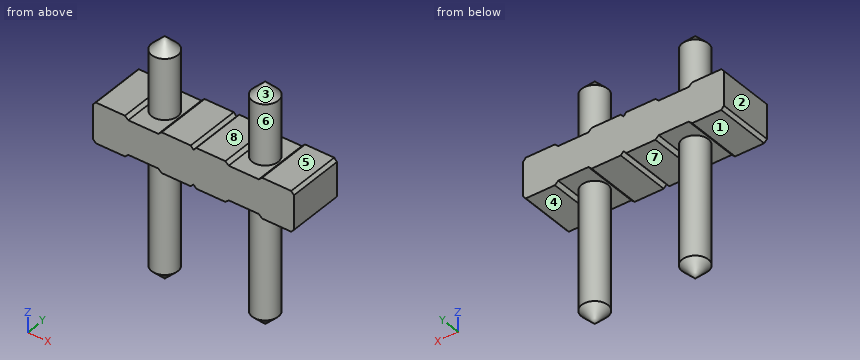
```python
from build123d import *

# Parameters (mm, degrees)
BOSS_EXTRUDE1_DEPTH = 1.4
SKETCH2_R           = 0.65
BOSS_EXTRUDE2_DEPTH = 5.9
BOSS_EXTRUDE3_START = 3
SKETCH3_R           = 0.65
BOSS_EXTRUDE3_DEPTH = 3
SKETCH5_R           = 0.65
BOSS_EXTRUDE4_DEPTH = 0.75
BOSS_EXTRUDE4_TAPER = 45


with BuildPart() as part:
    # Sketch1 → Boss-Extrude1 (new, symmetric)
    with BuildSketch(Plane(origin=(0, 0, 0), x_dir=(1, 0, 0), z_dir=(0, 1, 0))):
        Polygon((-2.5, -0.85), (-2.5, 0.85), (-2.362664546, 1), (-0.913832422, 1), (-0.75, 0.85), (0.75, 0.85), (0.913832422, 1), (2.362664546, 1), (2.5, 0.85), (2.5, -0.85), (2.362664546, -1), (0.913832422, -1), (0.75, -0.85), (-0.75, -0.85), (-0.913832422, -1), (-2.362664546, -1), align=None)
    extrude(amount=BOSS_EXTRUDE1_DEPTH, both=True)

    # Sketch2 → Boss-Extrude2 (add)
    with BuildSketch(Plane(origin=(0, 0, -0.85), x_dir=(-1, 0, 0), z_dir=(0, 0, -1))):
        with Locations(Location((0, 0, 0), (0, 0, 180))):
            Circle(SKETCH2_R)
    extrude(amount=BOSS_EXTRUDE2_DEPTH)

    # Sketch3 → Boss-Extrude3 (add)
    with BuildSketch(Plane.XY.offset(0.85).offset(BOSS_EXTRUDE3_START)):
        Circle(SKETCH3_R)
    extrude(amount=-BOSS_EXTRUDE3_DEPTH)

    # Sketch5 → Boss-Extrude4 (add)
    with BuildSketch(Plane.XY.offset(3.85)):
        Circle(SKETCH5_R)
    extrude(amount=BOSS_EXTRUDE4_DEPTH, taper=BOSS_EXTRUDE4_TAPER)

    # Boss-Extrude5 cone 1 section (through the dimple's axis) → Boss-Extrude5 (revolve)
    with BuildSketch(Plane(origin=(0, 0, -6.75), x_dir=(0, -1, 0), z_dir=(1, 0, 0))):
        Polygon((0, 0), (0.65, 0), (0, 0.65), align=None)
    revolve(axis=Axis((0, 0, -6.75), (0, 0, -1)))

    # Mirror1: part across plane


with BuildPart() as part_1:
    add(part.part)
    add(part.part.mirror(Plane(origin=(-2.5, 1.4, 0.85), x_dir=(0, 0, 1), z_dir=(1, 0, 0))))


solid = part_1.part
```
Can you work these out from the model? Positions are in its coordinate system, mm. Face numbers are marked on the shaded views. A direction names the side the tool comes from. Round coordinates to 2 decimals unless told otherwise and drop trailing zeros. Loops run counter-clockwise (first coordinate to the right, second up) from the corner with the lowest first, then second, coordinate; pieces in that order, holes last. Notation, with made-up numbers: M 70,85 L 94,85 A30 ccw 94,117 Z; hole C 52,66 d7. An arc over 180 degrees is marked long. Answer in a Markdown table with one row per item.
1. Thinking about a two-plate mould opening in X: for the marked faces 1, 2 and 3, which applies, pulls with the +X half, pulls with the -X half, needs draft (parallel to the pull), parting line crosses it, or undercut?
Established:
| item | result |
|---|---|
| face 1 | needs draft |
| face 2 | pulls with the -X half |
| face 3 | undercut |
2. I'm going to push flat-ended pins straight in: pin 1 Ø1.6 at (x, y) = (-2, 0.5) entering from +Z; pin 2 Ø1.6 at (x, y) = (-1.5, 0.5) entering from -Z; pin 3 Ø0.8 at (x, y) = (-5, -0.5) entering from -Z. Where does each tip first touch, or does it pass through?
Established:
| item | result |
|---|---|
| pin 1 | z = 1 |
| pin 2 | z = -1 |
| pin 3 | z = -7.3 |
3. On a 3-axis mill with a long thin cutter (end or side, diameter ignored), from which of +Z, -Z, +X, -X, +Y, -Y can I reach the whole of each face in a straight line? I mean the marked faces 4, 5, 6, 7 and 8. Say none if no direction works.
Established:
| item | result |
|---|---|
| face 4 | -Z, +X, +Y, -Y |
| face 5 | +Z, +X, +Y, -Y |
| face 6 | +Z |
| face 7 | -Z, +Y, -Y |
| face 8 | +Z, +Y, -Y |
4. If we section it at C-C, the plane x = -3.5: Please give me the cut outline in (y, z).
Established:
| item | result |
|---|---|
| outline | M -1.4,-1 L 1.4,-1 L 1.4,1 L -1.4,1 Z |
5. Please list where these lines run through material, in increasing order: line 1 (Z direction, x = -1.5, y = -0.05); line 2 (Z direction, x = -4.75, y = 1.05); line 3 (X direction, y = -0.5, z = -4.5). Write a range as from..to.
Established:
| item | result |
|---|---|
| line 1 | -1..1 |
| line 2 | -0.85..0.85 |
| line 3 | -5.42..-4.58, -0.42..0.42 |
6. If we section it at B-B, the plane z = -2: Please give me the cut outline in (x, y), plus the area to 3 significant figures.
Established:
| item | result |
|---|---|
| outline | C -5,0 d1.3; C 0,0 d1.3 |
| area | 2.65 mm² |
